The listing builds one solid part. Answer for the finished solid, in the listing's coordinates (mm). A direction names the side the tool comes from. Give positions to 0.01 mm unless a question says otherwise; leave off trailing zeros. Loops run counter-clockwise (first coordinate to the right, second up) from the corner with the lowest first, then second, coordinate; pieces in that order, holes last. Notation, with made-up numbers: (33, 0) - (85, 0) arc R6 cw to (85, 5) - close; hole circle Ø4 at (25, -22.75). An arc over 180 degrees is marked (long way). One line per item, written item: value. Start each with the question number.
from build123d import *

# Parameters (mm, degrees)
BOSS_EXTRUDE1_DEPTH = 25
BOSS_EXTRUDE3_DEPTH = 5
SKETCH6_R           = 7.5
BOSS_EXTRUDE4_DEPTH = 15
SKETCH7_R           = 4.05
CUT_EXTRUDE1_DEPTH  = 20
SKETCH8_R           = 2.5
CUT_EXTRUDE2_DEPTH  = 34.541019662


with BuildPart() as part:
    # Sketch2 → Boss-Extrude1 (new, symmetric)
    with BuildSketch(Plane(origin=(0, 0, 0), x_dir=(0, 0, -1), z_dir=(1, 0, 0))):
        Polygon((-3, 6.1), (3, 6.1), (3, 4.2), (5.3, 4.2), (5.3, 2.58), (2.8, 0), (-2.8, 0), (-5.3, 2.58), (-5.3, 4.2), (-3, 4.2), align=None)
    extrude(amount=BOSS_EXTRUDE1_DEPTH, both=True)

    # Sketch5 → Boss-Extrude3 (add)
    with BuildSketch(Plane(origin=(0, 6.1, 0), x_dir=(1, 0, 0), z_dir=(0, 1, 0))):
        with BuildLine():
            Line((8.306623863, -10), (-8.306623863, -10))
            ThreePointArc((-8.306623863, -10), (-13, 0), (-8.306623863, 10))
            Line((-8.306623863, 10), (8.306623863, 10))
            ThreePointArc((8.306623863, 10), (13, 0), (8.306623863, -10))
        make_face()
    extrude(amount=BOSS_EXTRUDE3_DEPTH)

    # Sketch6 → Boss-Extrude4 (add)
    with BuildSketch(Plane(origin=(0, 11.1, 0), x_dir=(1, 0, 0), z_dir=(0, 1, 0))):
        with Locations(Location((0, 0, 0), (0, 0, 270))):
            Circle(SKETCH6_R)
    extrude(amount=BOSS_EXTRUDE4_DEPTH)

    # Sketch7 → Cut-Extrude1 (cut)
    with BuildSketch(Plane(origin=(0, 26.1, 0), x_dir=(1, 0, 0), z_dir=(0, 1, 0))):
        with Locations(Location((0, 0, 0), (0, 0, 270))):
            Circle(SKETCH7_R)
    extrude(amount=-CUT_EXTRUDE1_DEPTH, mode=Mode.SUBTRACT)

    # Sketch8 → Cut-Extrude2 (cut, through all)
    with BuildSketch(Plane(origin=(0, 6.1, 0), x_dir=(1, 0, 0), z_dir=(0, 1, 0))):
        with Locations(Location((20, 0, 0), (0, 0, 270))):
            Circle(SKETCH8_R)
        with Locations(Location((-20, 0, 0), (0, 0, 270))):
            Circle(SKETCH8_R)
    extrude(amount=-CUT_EXTRUDE2_DEPTH, mode=Mode.SUBTRACT)


solid = part.part
1. Flat-ended cylindrical pins translate along their axes: pin 1 (3 mm diameter, centred on x = -8, y = 17.5, fed in from +Z); pin 2 (1.2 mm diameter, centred on x = 12, z = 4.5, fed in from +Y); pin 3 (4 mm diameter, centred on y = 18.5, z = -4.5, fed in from +X). Find the tip coordinate at first contact, or state that the pin passes through.
2. A cutting plane is placed at C-C (x = 0). Determine the outline of the cut face in (y, z), plus the area to 3 significant figures.
3. Find the intervals of material crossed by L1, parallel to X at y = 3, z = 0; L2, parallel to X at y = 18.75, z = 0; L3, parallel to X at y = 3, z = -2, in increasing order. Write a range as [from, to].
4. A cutting plane is placed at B-B (z = 0). Determine the outline of the cut face in (x, y).
5. Determine the mould class of faces 1 (the cylindrical face through (13, 9, 0)), 2 (the flat face through (-25, 3, 0)), 3 (the flat face through (0, 6.1, 0)) for opening direction Z: released by +Z, released by -Z, zero draft, split by the parting line, or undercut.
6. For faces 4 (the flat face through (0, 3, 5.3)), 5 (the flat face through (0, 5, -3)), 6 (the flat face through (0, 5, 3)), 7 (the flat face through (0, 3, -5.3)), determine the directions among +Z, -Z, +X, -X, +Y, -Y from which every point of the face is accessible in a straight line to the end or side of a thin tool.
7. A cutting plane is placed at A-A (x = 20). Determine the outline of the cut face in (y, z).
8. A cutting plane is placed at D-D (x = -14). Determine the outline of the cut face in (y, z).
Results below:
1. pin 1: stops at z = 3.74
1. pin 2: stops at y = 11.1
1. pin 3: stops at x = 7.07
2. outline: (0, -2.8) - (2.58, -5.3) - (4.2, -5.3) - (4.2, -3) - (6.1, -3) - (6.1, 3) - (4.2, 3) - (4.2, 5.3) - (2.58, 5.3) - (0, 2.8) - close; (6.1, -10) - (11.1, -10) - (11.1, -7.5) - (26.1, -7.5) - (26.1, -4.05) - (6.1, -4.05) - close; (6.1, 4.05) - (26.1, 4.05) - (26.1, 7.5) - (11.1, 7.5) - (11.1, 10) - (6.1, 10) - close
2. area: 212 mm^2
3. L1: x = [-25, -22.5], [-17.5, 17.5], [22.5, 25]
3. L2: x = [-7.5, -4.05], [4.05, 7.5]
3. L3: x = [-25, -21.5], [-18.5, 18.5], [21.5, 25]
4. outline: (-25, 0) - (-22.5, 0) - (-22.5, 6.1) - (-25, 6.1) - close; (-17.5, 0) - (17.5, 0) - (17.5, 6.1) - (13, 6.1) - (13, 11.1) - (7.5, 11.1) - (7.5, 26.1) - (4.05, 26.1) - (4.05, 6.1) - (-4.05, 6.1) - (-4.05, 26.1) - (-7.5, 26.1) - (-7.5, 11.1) - (-13, 11.1) - (-13, 6.1) - (-17.5, 6.1) - close; (22.5, 0) - (25, 0) - (25, 6.1) - (22.5, 6.1) - close
5. face 1: split by the parting line
5. face 2: zero draft
5. face 3: undercut
6. face 4: +Z, +X, -X, -Y
6. face 5: -Z, +X, -X
6. face 6: +Z, +X, -X
6. face 7: -Z, +X, -X, -Y
7. outline: (0, -2.8) - (2.58, -5.3) - (4.2, -5.3) - (4.2, -3) - (6.1, -3) - (6.1, -2.5) - (0, -2.5) - close; (0, 2.5) - (6.1, 2.5) - (6.1, 3) - (4.2, 3) - (4.2, 5.3) - (2.58, 5.3) - (0, 2.8) - close
8. outline: (0, -2.8) - (2.58, -5.3) - (4.2, -5.3) - (4.2, -3) - (6.1, -3) - (6.1, 3) - (4.2, 3) - (4.2, 5.3) - (2.58, 5.3) - (0, 2.8) - close
